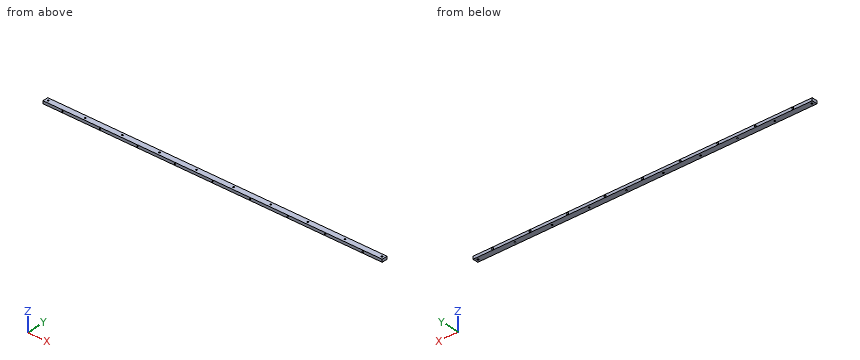
from build123d import *

# Parameters (mm, degrees)
SKETCH1_W           = 1549.4
SKETCH1_H           = 25.4
SKETCH1_R           = 3.429
BOSS_EXTRUDE1_DEPTH = 12.7
HOLE1_D             = 5.588
HOLE1_CBORE_D       = 8.636
HOLE1_CBORE_DEPTH   = 10.922
LPATTERN1_COUNT     = 9
LPATTERN1_PITCH     = 171.45
LPATTERN2_COUNT     = 9
LPATTERN2_PITCH     = 171.45


with BuildPart() as part:
    # Sketch1 → Boss-Extrude1 (new body)
    with BuildSketch(Plane.XY):
        with Locations((774.7, 12.7)):
            Rectangle(SKETCH1_W, SKETCH1_H)
        with Locations((12.7, 12.7)):
            Circle(SKETCH1_R, mode=Mode.SUBTRACT)
        with Locations((182.118, 12.7)):
            Circle(SKETCH1_R, mode=Mode.SUBTRACT)
        with Locations((351.536, 12.7)):
            Circle(SKETCH1_R, mode=Mode.SUBTRACT)
        with Locations((520.954, 12.7)):
            Circle(SKETCH1_R, mode=Mode.SUBTRACT)
        with Locations((690.372, 12.7)):
            Circle(SKETCH1_R, mode=Mode.SUBTRACT)
        with Locations((859.79, 12.7)):
            Circle(SKETCH1_R, mode=Mode.SUBTRACT)
        with Locations((1029.208, 12.7)):
            Circle(SKETCH1_R, mode=Mode.SUBTRACT)
        with Locations((1198.626, 12.7)):
            Circle(SKETCH1_R, mode=Mode.SUBTRACT)
        with Locations((1368.044, 12.7)):
            Circle(SKETCH1_R, mode=Mode.SUBTRACT)
        with Locations((1537.462, 12.7)):
            Circle(SKETCH1_R, mode=Mode.SUBTRACT)
    extrude(amount=-BOSS_EXTRUDE1_DEPTH)

    # Hole1 (through all)
    with Locations(Plane(origin=(88.9, 25.4, -6.35), x_dir=(0, 0, 1), z_dir=(0, 1, 0))):
        with Locations((0, 0)):
            hole1 = CounterBoreHole(HOLE1_D / 2, HOLE1_CBORE_D / 2, HOLE1_CBORE_DEPTH)

    # LPattern1: Hole1 ×9
    with Locations(*[(i * LPATTERN1_PITCH, 0, 0) for i in range(1, LPATTERN1_COUNT)]):
        add(hole1, mode=Mode.SUBTRACT)

    # Sketch5 → Hole2 (revolve, cut)
    with BuildSketch(Plane(origin=(88.9, 0, -6.35), x_dir=(0, 0, -1), z_dir=(1, 0, 0))):
        Polygon((0, 0), (0, 25.4), (2.794, 25.4), (2.794, 9.906), (2.54, 9.906), (2.54, 0), align=None)
    hole2 = revolve(axis=Axis((88.9, 110, -6.35), (0, -1, 0)), mode=Mode.SUBTRACT)

    # LPattern2: Hole2 ×9
    with Locations(*[(i * LPATTERN2_PITCH, 0, 0) for i in range(1, LPATTERN2_COUNT)]):
        add(hole2, mode=Mode.SUBTRACT)


solid = part.part
CAD build for the part. Positions are in the model's coordinates, mm. Give positions to 0.01 mm unless a question says otherwise; leave off trailing zeros. One line per question, with ' | ' between items. Start each with the question number.
1. Saw through at A-A on y = 20.5. State how many separate pieces and enclosed holes the cut face has, plus the area to 3 significant figures.
2. Probe L1, parallel to Z at x = 431.8, y = 23.25; L2, parallel to Z at x = 774.7, y = 4.5. List the from-to ranges inside material, lowest first. Write a range as from..to.
3. Flat gauge pins, fed straight in: pin 1 (3 mm diameter, centred on x = 616, z = -4, fed in from -Y); pin 2 (4.5 mm diameter, centred on x = 88.5, z = -7, fed in from +Y). Where does each tip first touch, or does it go through?
Result sheet:
1) separate pieces: 1 | enclosed holes: 9 | area: 19,200 mm^2
2) L1: z = -12.7..-10.67, -2.03..0 | L2: z = -12.7..-9.14, -3.56..0
3) pin 1: stops at y = 0 | pin 2: stops at y = 14.48
